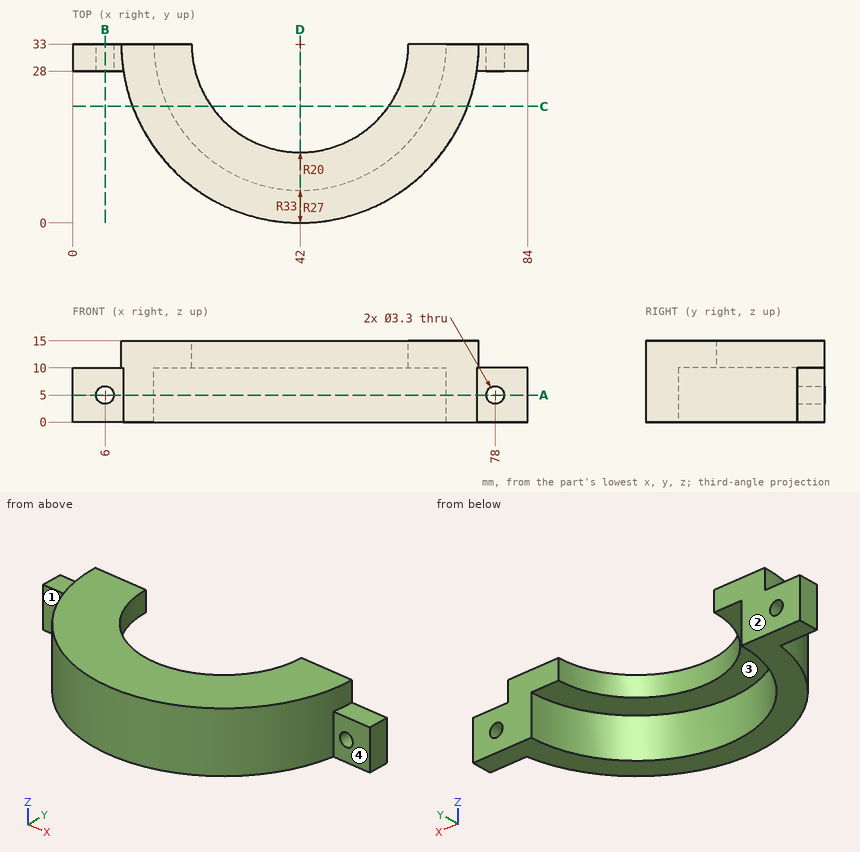
Verification items for this drawing (mm, ordinates from the low corner). A direction names the side the tool comes from. Give positions to 0.01 mm unless a question says otherwise; leave off trailing zeros. Loops run counter-clockwise (first coordinate to the right, second up) from the corner with the lowest first, then second, coordinate; pieces in that order, holes last.
1. Cross-section at C-C on y = 21.5. Record the cut outline in (x, z), and give its area (3 significant figures).
Derived:
outline: (11.07, 0) - (17.57, 0) - (17.57, 10) - (25.64, 10) - (25.64, 15) - (11.07, 15) - close; (58.36, 10) - (66.43, 10) - (66.43, 0) - (72.93, 0) - (72.93, 15) - (58.36, 15) - close
area: 276 mm2
2. Tool access check on the marked faces 1, 2, 3 and 4. Record the directions out of +Z, -Z, +X, -X, +Y, -Y that give a thin tool (end or side, any length) a straight path to the whole face; none if there is none.
Derived:
face 1: +Z, -Z, -X, -Y
face 2: +Z, -Z, +X, -X, +Y
face 3: -Z, +Y
face 4: +Z, -Z, +X, -Y
3. Cross-section at B-B on x = 6. Record the cut outline in (y, z), and give its area (3 significant figures).
Derived:
outline: (28, 0) - (33, 0) - (33, 3.35) - (28, 3.35) - close; (28, 6.65) - (33, 6.65) - (33, 10) - (28, 10) - close
area: 33.5 mm2
4. Cross-section at D-D on x = 42. Record the cut outline in (y, z), and give its area (3 significant figures).
Derived:
outline: (0, 0) - (6, 0) - (6, 10) - (13, 10) - (13, 15) - (0, 15) - close
area: 125 mm2
5. Material ranges on probe 1 along X at (y, z) = (30.05, 5); probe 2 along Z at (x, y) = (78, 31.6); probe 3 along X at (y, z) = (30.5, 5), recorded low to high.
Derived:
probe 1: x = 0 to 4.35, 7.65 to 15.16, 68.84 to 76.35, 79.65 to 84
probe 2: z = 0 to 3.35, 6.65 to 10
probe 3: x = 0 to 4.35, 7.65 to 15.12, 68.88 to 76.35, 79.65 to 84
6. Cross-section at A-A on z = 5. Record the cut outline in (x, y), and give its area (3 significant figures).
Derived:
outline: (0, 28) - (4.35, 28) - (4.35, 33) - (0, 33) - close; (7.65, 28) - (9.38, 28) arc R33 ccw to (74.62, 28) - (76.35, 28) - (76.35, 33) - (69, 33) arc R27 cw to (15, 33) - (7.65, 33) - close; (79.65, 28) - (84, 28) - (84, 33) - (79.65, 33) - close
area: 624 mm2
7. Go/stop test with flat-tipped pins: P1, Ø1.5, axis at y = 22, z = 5.5, coming from the -X side; P2, Ø2, axis at x = 30.5, y = 11, coming from the -Z side; P3, Ø4.5, axis at x = 4.5, z = 5, coming from the -Y side; P4, Ø2.5, axis at x = 6, z = 5, coming from the -Y side. Record where each tip stops, or that it passes through.
Derived:
P1: stops at x = 10.63
P2: stops at z = 10
P3: stops at y = 28
P4: passes through
